Can you work these out from the model? Positions are in its coordinate system, mm. A direction names the side the tool comes from. Round coordinates to 2 decimals unless told otherwise and drop trailing zeros. Loops run counter-clockwise (first coordinate to the right, second up) from the corner with the lowest first, then second, coordinate; pieces in that order, holes last. Notation, with made-up numbers: (-13, 78) - (9, 78) arc R31 cw to (9, 108) - close; hole circle Ø5 at (-16, 45.5). An arc over 180 degrees is marked (long way). Answer as CSV lines item,"result".
Autodesk Inventor part; units mm, degrees
ref_plane "YZ Plane" through (0, 0, 0) normal (1, 0, 0) x (0, 1, 0)
ref_plane "XZ Plane" through (0, 0, 0) normal (0, 1, 0) x (-1, 0, 0)
ref_plane "XY Plane" through (0, 0, 0) normal (0, 0, 1) x (1, 0, 0)
ref_plane "작업 평면1" through (0, 0, 0) normal (0, 0, 1) x (1, 0, 0)
sketch "스케치1" plane through (0, 0, 0) normal (0, 0, 1) x (1, 0, 0)
  circle A0 centre (-20, 40) radius 1.35
  circle A1 centre (20, 40) radius 1.35
  line L0 (6.05, 36.95) -> (-6.05, 36.95)
  line L1 (-6.05, 36.95) -> (-6.05, 43.05)
  line L2 (-6.05, 43.05) -> (6.05, 43.05)
  line L3 (6.05, 43.05) -> (6.05, 36.95)
  line L4 (-37, 6) -> (-37, 45)
  line L5 (-37, 6) -> (-43, 6)
  line L6 (-43, 6) -> (-43, -6)
  line L7 (-43, -6) -> (-37, -6)
  line L8 (-37, -6) -> (-37, -35)
  line L9 (-37, -35) -> (37, -35)
  line L10 (37, -35) -> (37, -6)
  line L11 (37, -6) -> (43, -6)
  line L12 (43, -6) -> (43, 6)
  line L13 (43, 6) -> (37, 6)
  line L14 (37, 6) -> (37, 45)
  line L15 (-37, 45) -> (37, 45)
  circle A2 centre (-28.8, -30.8) radius 1.35
  circle A3 centre (28.8, -30.8) radius 1.35
  circle A4 centre (28.8, 30.8) radius 1.35
  circle A5 centre (-20.8, -30.8) radius 1.6
  circle A6 centre (-20.8, 30.8) radius 1.6
  circle A7 centre (20.8, -30.8) radius 1.6
  circle A8 centre (20.8, 30.8) radius 1.6
  circle A9 centre (-28.8, 30.8) radius 1.35
  line L16 (31.1, -8.4) -> (31.1, -13.6)
  line L17 (31.1, -13.6) -> (28.9, -13.6)
  line L18 (28.9, -13.6) -> (28.9, -8.4)
  line L19 (28.9, -8.4) -> (31.1, -8.4)
  line L20 (-31.1, -8.4) -> (-28.9, -8.4)
  line L21 (-28.9, -8.4) -> (-28.9, -13.6)
  line L22 (-28.9, -13.6) -> (-31.1, -13.6)
  line L23 (-31.1, -13.6) -> (-31.1, -8.4)
  line L24 (-31.1, 13.6) -> (-28.9, 13.6)
  line L25 (-28.9, 13.6) -> (-28.9, 8.4)
  line L26 (-28.9, 8.4) -> (-31.1, 8.4)
  line L27 (-31.1, 8.4) -> (-31.1, 13.6)
  line L28 (28.9, 13.6) -> (31.1, 13.6)
  line L29 (31.1, 13.6) -> (31.1, 8.4)
  line L30 (31.1, 8.4) -> (28.9, 8.4)
  line L31 (28.9, 8.4) -> (28.9, 13.6)
  line L32 (37, 37) -> (-37, 37)
  line L33 (-37, 37) -> (-37, 43)
  line L34 (-37, 43) -> (37, 43)
  line L35 (37, 43) -> (37, 37)
  line L36 (37, 37) -> (-37, 43) construction
  line L37 (-37, 37) -> (37, 43) construction
  point P0 (0, 0)
  point P1 (0, 40)
  dimension "d0" = 74
  dimension "d1" = 6
extrude "돌출1" add sketch "스케치1" along normal blind 50 contours L32 L1 L34 L3 | L3 L34 L14 L32 | L32 L4 L34 L1
sketch "스케치2" plane through (0, 0, 50) normal (0, 0, 1) x (1, 0, 0)
  line L0 (6.05, 43) -> (-6.05, 43)
  line L1 (-6.05, 43) -> (-6.05, 37)
  line L2 (-6.05, 37) -> (6.05, 37)
  line L3 (6.05, 37) -> (6.05, 43)
  line L4 (6.05, 43) -> (-6.05, 37) construction
  line L5 (-6.05, 43) -> (6.05, 37) construction
  point P0 (0, 0)
  point P1 (0, 40)
  dimension "d4" = 12.1
  dimension "d5" = 6
extrude "돌출2" cut sketch "스케치2" against normal blind 6.1
sketch "스케치3" plane through (0, 0, 0) normal (0, 0, -1) x (-1, 0, 0)
  line L0 (-6, 37) -> (6, 37)
  line L1 (6, 37) -> (6, 43)
  line L2 (6, 43) -> (-6, 43)
  line L3 (-6, 43) -> (-6, 37)
  line L4 (-6, 37) -> (6, 43) construction
  line L5 (6, 37) -> (-6, 43) construction
  point P0 (0, 0)
  point P1 (0, 40)
  dimension "d8" = 12
  dimension "d9" = 6
extrude "돌출3" add sketch "스케치3" along normal blind 6
sketch "스케치4" plane through (37, 43, 50) normal (0, 1, 0) x (1, 0, 0)
  line L0 (-58.35, 0) -> (-58.35, 50)
  line L1 (-55.65, 0) -> (-55.65, 50)
  line L2 (-18.35, 0) -> (-18.35, 50)
  line L3 (-15.65, 0) -> (-15.65, 50)
  line L4 (-15.65, 35) -> (-18.35, 35)
  line L5 (-55.65, 35) -> (-58.35, 35)
  line L6 (-14.4, 36.1) -> (-19.6, 33.9) construction
  line L7 (-19.6, 36.1) -> (-14.4, 33.9) construction
  line L8 (-54.4, 36.1) -> (-59.6, 36.1)
  line L9 (-59.6, 36.1) -> (-59.6, 33.9)
  line L10 (-59.6, 33.9) -> (-54.4, 33.9)
  line L11 (-54.4, 33.9) -> (-54.4, 36.1)
  line L12 (-54.4, 36.1) -> (-59.6, 33.9) construction
  line L13 (-59.6, 36.1) -> (-54.4, 33.9) construction
  circle A0 centre (-9, 3) radius 1.35
  circle A1 centre (-65, 3) radius 1.35
  line L14 (-14.4, 46.1) -> (-19.6, 46.1)
  line L15 (-19.6, 46.1) -> (-19.6, 43.9)
  line L16 (-19.6, 43.9) -> (-14.4, 43.9)
  line L17 (-14.4, 43.9) -> (-14.4, 46.1)
  line L18 (-14.4, 46.1) -> (-19.6, 43.9) construction
  line L19 (-19.6, 46.1) -> (-14.4, 43.9) construction
  line L20 (-54.4, 46.1) -> (-59.6, 46.1)
  line L21 (-59.6, 46.1) -> (-59.6, 43.9)
  line L22 (-59.6, 43.9) -> (-54.4, 43.9)
  line L23 (-54.4, 43.9) -> (-54.4, 46.1)
  line L24 (-54.4, 46.1) -> (-59.6, 43.9) construction
  line L25 (-59.6, 46.1) -> (-54.4, 43.9) construction
  point P0 (-37, 50)
  point P1 (-17, 35)
  point P2 (-57, 35)
  point P3 (-17, 45)
  point P4 (-57, 45)
  dimension "d12" = 5.2
  dimension "d13" = 2.2
  dimension "d14" = 5.2
  dimension "d15" = 2.2
  dimension "d16" = 2.7
  dimension "d17" = 2.7
  dimension "d20" = 5.2
  dimension "d21" = 2.2
  dimension "d22" = 5.2
  dimension "d23" = 2.2
extrude "돌출5" cut sketch "스케치4" against normal blind 50 contours L22 L21 L20 L0 | L0 L20 L1 L22 | L1 L20 L23 L22 | L16 L15 L14 L2 | L2 L14 L3 L16 | L3 L14 L17 L16 | A0 | A1
sketch "스케치5" plane through (-37, 37, 0) normal (-1, 0, 0) x (0, 0, 1)
  line L0 (50, 6) -> (0, 6)
  line L1 (0, 6) -> (0, 0)
  line L2 (0, 0) -> (50, 0)
  line L3 (50, 0) -> (50, 6)
  point P0 (0, -37)
extrude "돌출6" add sketch "스케치5" along normal blind 6
sketch "스케치6" plane through (37, 37, 0) normal (1, 0, 0) x (0, 0, -1)
  line L0 (-50, 0) -> (0, 0)
  line L1 (0, 0) -> (0, 6)
  line L2 (0, 6) -> (-50, 6)
  line L3 (-50, 6) -> (-50, 0)
  point P0 (0, -37)
  dimension "d28" = 6
extrude "돌출7" add sketch "스케치6" along normal blind 6
sketch "스케치7" plane through (-6.05, 43, 43.9) normal (0, 1, 0) x (1, 0, 0)
  circle A0 centre (26.05, 13) radius 5
  circle A1 centre (-13.95, 13) radius 5
  line L0 (21.05, 28.5) -> (-8.95, 28.5)
  line L1 (-8.95, 28.5) -> (-8.95, 31.5)
  line L2 (-8.95, 31.5) -> (21.05, 31.5)
  line L3 (21.05, 31.5) -> (21.05, 28.5)
  line L4 (21.05, 28.5) -> (-8.95, 31.5) construction
  line L5 (-8.95, 28.5) -> (21.05, 31.5) construction
  point P0 (6.05, 43.9)
  point P1 (6.05, 30)
  dimension "d31" = 10
  dimension "d32" = 10
  dimension "d35" = 3
extrude "돌출9" cut sketch "스케치7" against normal blind 10
sketch "스케치8" plane through (-6.05, 43, 43.9) normal (0, 1, 0) x (1, 0, 0)
  line L0 (-8.95, 28.5) -> (-8.95, 31.5)
  line L1 (-8.95, 31.5) -> (21.05, 31.5)
  line L2 (21.05, 31.5) -> (21.05, 28.5)
  line L3 (21.05, 28.5) -> (-8.95, 28.5)
  circle A0 centre (-13.95, 13) radius 5
  circle A1 centre (26.05, 13) radius 5
  circle A2 centre (-21.95, -3.1) radius 1.35
  line L4 (-16.55, 37.8) -> (-16.55, 40)
  line L5 (-16.55, 40) -> (-11.35, 40)
  line L6 (-11.35, 40) -> (-11.35, 37.8)
  line L7 (-11.35, 37.8) -> (-16.55, 37.8)
  circle A3 centre (34.05, -3.1) radius 1.35
  line L8 (23.45, 40) -> (28.65, 40)
  line L9 (28.65, 40) -> (28.65, 37.8)
  line L10 (28.65, 37.8) -> (23.45, 37.8)
  line L11 (23.45, 37.8) -> (23.45, 40)
  line L12 (0, -6.1) -> (0, 0)
  line L13 (0, 0) -> (12.1, 0)
  line L14 (12.1, 0) -> (12.1, -6.1)
  line L15 (12.1, -6.1) -> (49.05, -6.1)
  line L16 (49.05, 43.9) -> (49.05, -6.1)
  line L17 (12.05, 43.9) -> (49.05, 43.9)
  line L18 (12.05, 43.9) -> (12.05, 49.9)
  line L19 (0.05, 49.9) -> (12.05, 49.9)
  line L20 (0.05, 43.9) -> (0.05, 49.9)
  line L21 (0.05, 43.9) -> (-36.95, 43.9)
  line L22 (-36.95, -6.1) -> (-36.95, 43.9)
  line L23 (0, -6.1) -> (-36.95, -6.1)
  circle A4 centre (-33.95, -0.1) radius 1.35
  circle A5 centre (46.05, 0) radius 1.35
  point P0 (6.05, 43.9)
  dimension "d38" = 2.7
  dimension "d41" = 2.7
extrude "돌출11" cut sketch "스케치8" against normal blind 10 contours A4 | A5
sketch "스케치9" plane through (-6.05, 43, 43.9) normal (0, 1, 0) x (1, 0, 0)
  line L0 (0, 0) -> (12.1, 0)
  line L1 (12.1, 0) -> (12.1, -6.1)
  line L2 (0, -6.1) -> (0, 0)
  circle A0 centre (12.1, 0) radius 1
  circle A1 centre (0, 0) radius 1
  point P0 (6.05, 43.9)
  point P1 (12.1, -1)
  point P2 (11.1, 0)
  dimension "d44" = 2
  dimension "d45" = 2
extrude "돌출12" cut sketch "스케치9" against normal blind 10 contours L2 A1 L0 | L0 A1 L2 | A0 L1 L0 picked at (11.443, 0.0798)
properties part number "front of head" material "PMMA 플라스틱"
Q1. If I drill on line 1 along X through (y, z) = (38.5, 30.9); line 2 along X through (y, z) = (40, 1.5); line 3 along X through (y, z) = (39.75, 46.5), over which ranges is the centre line in solid material (lowest first)? Write a range as [from, to].
Checks:
line 1,"[-43, -25], [-15, 15], [25, 43]"
line 2,"[-43, -21.35], [-18.65, 18.65], [21.35, 43]"
line 3,"[-43, -29.25], [-26.75, -21.33], [-18.67, -6.05], [6.05, 18.67], [21.33, 26.75], [29.25, 43]"
Q2. I'm going to push flat-ended pins straight in: pin 1 Ø3 at (y, z) = (40.5, -2.5) entering from -X; pin 2 Ø3 at (x, y) = (20, 40) entering from -Z; pin 3 Ø3 at (x, z) = (-28, 47) entering from -Y. Where does each tip first touch, or does it pass through?
Checks:
pin 1,"x = -6"
pin 2,"z = 0"
pin 3,"y = 37"
Q3. Imagine slicing it at A-A (z = 5). Write out the boundary of the cut face in (x, y), then the cut area to 3 significant figures.
Checks:
outline,"(-43, 37) - (-22.6, 37) - (-22.6, 43) - (-43, 43) - close; (-17.4, 37) - (17.4, 37) - (17.4, 43) - (-17.4, 43) - close; (22.6, 37) - (43, 37) - (43, 43) - (22.6, 43) - close"
area,"454 mm²"
Q4. We'd pull the mould along Y, two halves only. Please class faces 5 (the flat face through (43, 40, 25)), 6 (the cylindrical face through (20.62, 41.2, 42.76)): pulls with the +Y half, pulls with the -Y half, needs draft (parallel to the pull), parting line crosses it, or undercut.
Checks:
face 5,"needs draft"
face 6,"undercut"
Q5. Imagine slicing it at B-B (x = -20). Write out the boundary of the cut face in (y, z), then the cut area to 3 significant figures.
Checks:
outline,"(37, 0) - (38.65, 0) - (38.65, 3.9) - (37, 3.9) - close; (37, 6.1) - (38.65, 6.1) - (38.65, 25.9) - (37, 25.9) - close; (37, 35.9) - (38.65, 35.9) - (38.65, 50) - (37, 50) - close; (41.35, 0) - (43, 0) - (43, 3.9) - (41.35, 3.9) - close; (41.35, 6.1) - (43, 6.1) - (43, 25.9) - (41.35, 25.9) - close; (41.35, 35.9) - (43, 35.9) - (43, 50) - (41.35, 50) - close"
area,"125 mm²"
Q6. On a 3-axis mill with a long thin cutter (end or side, diameter ignored), from which of +Z, -Z, +X, -X, +Y, -Y can I reach the whole of each face in a straight line? I mean faces 1 (the flat face through (0, 40, 43.9)), 2 (the flat face through (0, 40, 12.4)), 3 (the flat face through (-24, 40, 0)), 4 (the flat face through (6, 40, -3)). Say none if no direction works.
Checks:
face 1,"+Z, +Y, -Y"
face 2,"+Y, -Y"
face 3,"-Z, -X, +Y, -Y"
face 4,"-Z, +X, +Y, -Y"
Q7. Imagine slicing it at C-C (z = 47). Write out the boundary of the cut face in (x, y).
Checks:
outline,"(-43, 37) - (-29.35, 37) - (-29.35, 43) - (-43, 43) - close; (-26.65, 37) - (-6.05, 37) - (-6.05, 43) - (-26.65, 43) - close; (6.05, 37) - (26.65, 37) - (26.65, 43) - (6.05, 43) - close; (29.35, 37) - (43, 37) - (43, 43) - (29.35, 43) - close; hole circle Ø2.7 at (-20, 40); hole circle Ø2.7 at (20, 40)"
Q8. Imagine slicing it at D-D (x = -0.5). Write out the boundary of the cut face in (y, z), then the cut area to 3 significant figures.
Checks:
outline,"(37, -6) - (43, -6) - (43, 12.4) - (37, 12.4) - close; (37, 15.4) - (43, 15.4) - (43, 43.9) - (37, 43.9) - close"
area,"281 mm²"
